```python
from build123d import *

# Parameters (mm, degrees)
SKETCH1_R           = 3.4
BOSS_EXTRUDE1_DEPTH = 350


with BuildPart() as part:
    # Sketch1 → Boss-Extrude1 (new body)
    with BuildSketch(Plane(origin=(0, 0, 0), x_dir=(1, 0, 0), z_dir=(0, 1, 0))):
        with BuildLine():
            Line((5.8, 4.385786438), (5.8, -4.385786438))
            Line((5.8, -4.385786438), (9.664213562, -8.25))
            Line((9.664213562, -8.25), (12.8, -8.25))
            Line((12.8, -8.25), (12.8, -4.1))
            Line((12.8, -4.1), (15, -4.1))
            Line((15, -4.1), (15, -12.5))
            ThreePointArc((15, -12.5), (14.267766953, -14.267766953), (12.5, -15))
            Line((12.5, -15), (4.1, -15))
            Line((4.1, -15), (4.1, -12.8))
            Line((4.1, -12.8), (8.25, -12.8))
            Line((8.25, -12.8), (8.25, -9.664213562))
            Line((8.25, -9.664213562), (4.385786438, -5.8))
            Line((4.385786438, -5.8), (-4.385786438, -5.8))
            Line((-4.385786438, -5.8), (-8.25, -9.664213562))
            Line((-8.25, -9.664213562), (-8.25, -12.8))
            Line((-8.25, -12.8), (-4.1, -12.8))
            Line((-4.1, -12.8), (-4.1, -15))
            Line((-4.1, -15), (-12.5, -15))
            ThreePointArc((-12.5, -15), (-14.267766953, -14.267766953), (-15, -12.5))
            Line((-15, -12.5), (-15, -4.1))
            Line((-15, -4.1), (-12.8, -4.1))
            Line((-12.8, -4.1), (-12.8, -8.25))
            Line((-12.8, -8.25), (-9.664213562, -8.25))
            Line((-9.664213562, -8.25), (-5.8, -4.385786438))
            Line((-5.8, -4.385786438), (-5.8, 4.385786438))
            Line((-5.8, 4.385786438), (-9.664213562, 8.25))
            Line((-9.664213562, 8.25), (-12.8, 8.25))
            Line((-12.8, 8.25), (-12.8, 4.1))
            Line((-12.8, 4.1), (-15, 4.1))
            Line((-15, 4.1), (-15, 12.5))
            ThreePointArc((-15, 12.5), (-14.267766953, 14.267766953), (-12.5, 15))
            Line((-12.5, 15), (-4.1, 15))
            Line((-4.1, 15), (-4.1, 12.8))
            Line((-4.1, 12.8), (-8.25, 12.8))
            Line((-8.25, 12.8), (-8.25, 9.664213562))
            Line((-8.25, 9.664213562), (-4.385786438, 5.8))
            Line((-4.385786438, 5.8), (4.385786438, 5.8))
            Line((4.385786438, 5.8), (8.25, 9.664213562))
            Line((8.25, 9.664213562), (8.25, 12.8))
            Line((8.25, 12.8), (4.1, 12.8))
            Line((4.1, 12.8), (4.1, 15))
            Line((4.1, 15), (12.5, 15))
            ThreePointArc((12.5, 15), (14.267766953, 14.267766953), (15, 12.5))
            Line((15, 12.5), (15, 4.1))
            Line((15, 4.1), (12.8, 4.1))
            Line((12.8, 4.1), (12.8, 8.25))
            Line((12.8, 8.25), (9.664213562, 8.25))
            Line((9.664213562, 8.25), (5.8, 4.385786438))
        make_face()
        Circle(SKETCH1_R, mode=Mode.SUBTRACT)
    extrude(amount=BOSS_EXTRUDE1_DEPTH)


solid = part.part
```
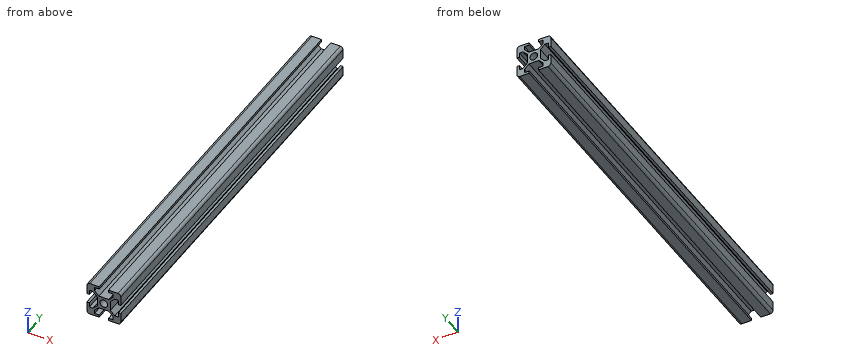
CAD build for the part. Positions are in the model's coordinates, mm. Coordinates: 2 decimals unless noted, no trailing zeros. Write each loop counter-clockwise with the first axis right and the second up, starting at its lowest first coordinate (ties: lowest second). Pieces come first, ordered by that corner, then holes. Notation, with made-up numbers: (-23, 55.5) -> (30, 55.5) arc R16 cw to (30, 79.5) -> close; hole circle Ø6 at (24.5, 29). An arc over 180 degrees is marked (long way). Use CSV: the item, a comma, the result in double quotes. Start each with the question number.
Item 1: Drop flat-ended pins along their axis: P1, Ø1.1, axis at y = 211.5, z = -13.5, coming from the -X side; P2, Ø7, axis at y = 96, z = 0.5, coming from the -X side; P3, Ø2.5, axis at y = 181, z = 0, coming from the +X side. Give the stop position or say it passes through.
Item 2: Band-saw the part on B-B, the plane x = 0. Write the cut outline in (y, z).
Item 3: Band-saw the part on A-A, the plane z = 0. Write the cut outline in (x, y).
Item 4: Wall check: probe 1 along Z at (x, y) = (10.25, 55.5); probe 2 along X at (y, z) = (151, 0). Give the ranges that are in metal, low to high.
Response values:
1,P1,"stops at x = -14.96"
1,P2,"stops at x = -5.8"
1,P3,"stops at x = 5.8"
2,outline,"(0, -5.8) -> (350, -5.8) -> (350, -3.4) -> (0, -3.4) -> close; (0, 3.4) -> (350, 3.4) -> (350, 5.8) -> (0, 5.8) -> close"
3,outline,"(-5.8, 0) -> (-3.4, 0) -> (-3.4, 350) -> (-5.8, 350) -> close; (3.4, 0) -> (5.8, 0) -> (5.8, 350) -> (3.4, 350) -> close"
4,probe 1,"z = -15 to -8.25, 8.25 to 15"
4,probe 2,"x = -5.8 to -3.4, 3.4 to 5.8"
